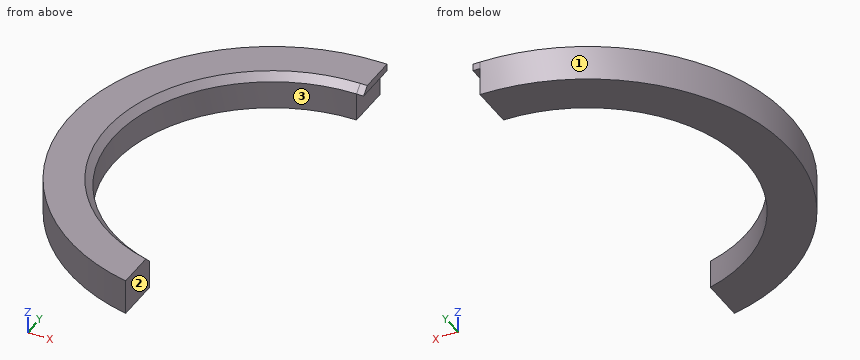
```python
from build123d import *

# Parameters (mm, degrees)
SKETCH1_R           = 57.5
SKETCH1_R_2         = 45
BOSS_EXTRUDE1_DEPTH = 10
CUT_EXTRUDE2_DEPTH  = 10
SKETCH3_W           = 124.113144638
SKETCH3_H           = 66.876500266
CUT_EXTRUDE3_DEPTH  = 10
CUT_EXTRUDE4_START  = -2
SKETCH5_R           = 4
CUT_EXTRUDE4_DEPTH  = 3
BOSS_EXTRUDE2_DEPTH = 2


with BuildPart() as part:
    # Sketch1 → Boss-Extrude1 (new body)
    with BuildSketch(Plane(origin=(0, 0, 0), x_dir=(0, 1, 0), z_dir=(0, 0, 1))):
        with Locations(Location((0, 0, 0), (0, 0, 270))):
            Circle(SKETCH1_R)
        with Locations(Location((0, 0, 0), (0, 0, 270))):
            Circle(SKETCH1_R_2, mode=Mode.SUBTRACT)
    extrude(amount=BOSS_EXTRUDE1_DEPTH)

    # Sketch2 → Cut-Extrude2 (cut)
    with BuildSketch(Plane(origin=(0, 0, 0), x_dir=(1, 0, 0), z_dir=(0, 0, -1))):
        with BuildLine():
            Line((11.650511373, 56.659857386), (11.650511373, 43.46568284))
            add(Edge.make_bspline(
                [(11.650511373, 43.46568284), (-0.679246558, 46.406413024), (-11.650511373, 43.46568284)],
                knots=[0, 0, 0, 0.575547458, 0.575547458, 0.575547458], degree=2))
            Line((-11.650511373, 43.46568284), (-11.650511373, 56.659857386))
            ThreePointArc((-11.650511373, 56.659857386), (0, 57.845257837), (11.650511373, 56.659857386))
        make_face()
    extrude(amount=-CUT_EXTRUDE2_DEPTH, mode=Mode.SUBTRACT)

    # Chamfer1: read off the stored shape, not the designer's step
    # Chamfer1 outline → Chamfer1 (revolve, cut)
    with BuildSketch(Plane.XZ):
        Polygon((45, 10.000000111), (45, 8), (47.000000111, 10.000000111), align=None)
    revolve(axis=Axis((0, 0, 0), (0, 0, 1)), mode=Mode.SUBTRACT)

    # Sketch3 → Cut-Extrude3 (cut)
    with BuildSketch(Plane(origin=(0, 0, 0), x_dir=(0, 1, 0), z_dir=(0, 0, 1))):
        with Locations((4.641630902, -33.438250133)):
            Rectangle(SKETCH3_W, SKETCH3_H)
    extrude(amount=CUT_EXTRUDE3_DEPTH, mode=Mode.SUBTRACT)

    # Sketch5 → Cut-Extrude4 (cut)
    with BuildSketch(Plane(origin=(0, 0, 0), x_dir=(1, 0, 0), z_dir=(0, 0, -1)).offset(CUT_EXTRUDE4_START)):
        with Locations(Location((-6, -51.25, 0), (0, 0, 180))):
            Circle(SKETCH5_R)
    extrude(amount=-CUT_EXTRUDE4_DEPTH, mode=Mode.SUBTRACT)

    # Sketch6 → Boss-Extrude2 (add)
    with BuildSketch(Plane.YZ):
        Polygon((45, 8), (47, 10), (57.5, 10), (57.5, 8), align=None)
    extrude(amount=BOSS_EXTRUDE2_DEPTH)


solid = part.part
```
Input: part model. Units: mm. Frame: model coordinates. Face numbers are marked on the shaded views. Give positions to 0.01 mm unless a question says otherwise; leave off trailing zeros. Order: outer loops, then holes, each group sorted by start corner. A loop starts at its lowest first (then second) coordinate and runs counter-clockwise, first axis right, second up.
1. Cut plane B-B (z = 6.75). Return loops of the section in (x, y), and give its area (3 significant figures).
Computed:
outline: (-11.65, -56.31) - (-11.65, -43.47) arc R45 cw to (0, 45) - (0, 57.5) arc R57.5 ccw to start
area: 1,870 mm2
2. Line query: probe 1 along Y at (x, z) = (-6, 2.95); probe 2 along Y at (x, z) = (-19, 4); probe 3 along X at (y, z) = (-11.5, 8). Output: solid intervals per line, ascending.
Computed:
probe 1: y = 44.6 to 47.25, 55.25 to 57.19
probe 2: y = -54.27 to -40.79, 40.79 to 54.27
probe 3: x = -56.34 to -43.51
3. Cut plane A-A (y = 51.25). Return loops of the section in (x, z).
Computed:
outline: (-26.07, 0) - (0, 0) - (0, 8) - (2, 8) - (2, 10) - (-26.07, 10) - close; hole (-10, 2) - (-2, 2) - (-2, 5) - (-10, 5) - close
4. Pin query (flat end, axial travel): pin 1 Ø1.6 at (x, y) = (1, 48.5) entering from -Z; pin 2 Ø5 at (y, z) = (3, 6.5) entering from +X; pin 3 Ø1.5 at (x, y) = (-27.5, 37) entering from +Z. Return the tip coordinate at first contact, or that it passes through.
Computed:
pin 1: stops at z = 8
pin 2: stops at x = -44.66
pin 3: stops at z = 9.85
5. Draft query along Y for the marked faces 1, 2 and 3. Return one class per face: released by +Y, released by -Y, zero draft, split by the parting line, or undercut.
Computed:
face 1: split by the parting line
face 2: zero draft
face 3: undercut
